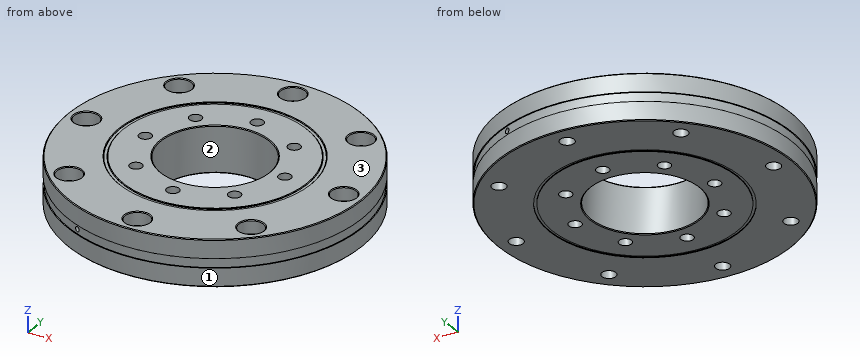
from build123d import *

# Parameters (mm, degrees)
BOSS_EXTRUDE1_DEPTH          = 7.5
BOSS_EXTRUDE1_DEPTH_BACK     = 7.5
SKETCH4_R                    = 2
CIRPATTERN1_COUNT            = 8
BOSS_EXTRUDE4_DEPTH          = 7.5
BOSS_EXTRUDE4_DEPTH_BACK     = 7.5
SKETCH9_R                    = 47.5
SKETCH9_R_2                  = 17.5
SKETCH10_R                   = 4
CUT_EXTRUDE1_DEPTH           = 4.4
SKETCH11_R                   = 2.25
CUT_EXTRUDE2_DEPTH           = 69.82949949
CHAMFER2_SIZE                = 0.25
CHAMFER1_SIZE                = 0.25
CIRPATTERN2_COUNT            = 8
CHAMFER2_OF_CIRPATTERN2_SIZE = 0.25
SKETCH12_W                   = 0.25
SKETCH12_H                   = 0.9
SKETCH12_W_2                 = 3
SKETCH12_H_2                 = 0.3
SKETCH13_W                   = 0.825
SKETCH13_H                   = 17.2
CIRPATTERN3_COUNT            = 2
CHAMFER3_SIZE                = 0.2


with BuildPart() as part:
    # Sketch4 → Boss-Extrude1 (new, two sides: drawn at the far end of the back side and taken through both)
    with BuildSketch(Plane.XY.offset(-BOSS_EXTRUDE1_DEPTH_BACK)):
        with Locations((0, 22.5)):
            Circle(SKETCH4_R)
    extrude(amount=BOSS_EXTRUDE1_DEPTH + BOSS_EXTRUDE1_DEPTH_BACK)

    # Boss-Extrude2 cone 1 section (through the dimple's axis) → Boss-Extrude2 (revolve)
    with BuildSketch(Plane(origin=(0, 22.5, 7.5), x_dir=(0, -1, 0), z_dir=(1, 0, 0))):
        Polygon((0, 0), (2, 0), (0, 2), align=None)
    revolve(axis=Axis((0, 22.5, 7.5), (0, 0, -1)))

    # Boss-Extrude3 cone 1 section (through the dimple's axis) → Boss-Extrude3 (revolve)
    with BuildSketch(Plane(origin=(0, 22.5, -7.5), x_dir=(0, 1, 0), z_dir=(1, 0, 0))):
        Polygon((0, 0), (2, 0), (0, 2), align=None)
    revolve(axis=Axis((0, 22.5, -7.5), (0, 0, 1)))


with BuildPart() as cirpattern1_1:
    # CirPattern1: pattern copy
    add(part.part.rotate(Axis((0, 0, 0), (0, 0, 1)), 1 * 360 / CIRPATTERN1_COUNT))


with BuildPart() as cirpattern1_2:
    # CirPattern1: pattern copy
    add(part.part.rotate(Axis((0, 0, 0), (0, 0, 1)), 2 * 360 / CIRPATTERN1_COUNT))


with BuildPart() as cirpattern1_3:
    # CirPattern1: pattern copy
    add(part.part.rotate(Axis((0, 0, 0), (0, 0, 1)), 3 * 360 / CIRPATTERN1_COUNT))


with BuildPart() as cirpattern1_4:
    # CirPattern1: pattern copy
    add(part.part.rotate(Axis((0, 0, 0), (0, 0, 1)), 4 * 360 / CIRPATTERN1_COUNT))


with BuildPart() as cirpattern1_5:
    # CirPattern1: pattern copy
    add(part.part.rotate(Axis((0, 0, 0), (0, 0, 1)), 5 * 360 / CIRPATTERN1_COUNT))


with BuildPart() as cirpattern1_6:
    # CirPattern1: pattern copy
    add(part.part.rotate(Axis((0, 0, 0), (0, 0, 1)), 6 * 360 / CIRPATTERN1_COUNT))


with BuildPart() as cirpattern1_7:
    # CirPattern1: pattern copy
    add(part.part.rotate(Axis((0, 0, 0), (0, 0, 1)), 7 * 360 / CIRPATTERN1_COUNT))


with BuildPart() as body_9:
    # Sketch9 → Boss-Extrude4 (new, two sides: drawn at the far end of the back side and taken through both)
    with BuildSketch(Plane.XY.offset(-BOSS_EXTRUDE4_DEPTH_BACK)):
        Circle(SKETCH9_R)
        Circle(SKETCH9_R_2, mode=Mode.SUBTRACT)
    extrude(amount=BOSS_EXTRUDE4_DEPTH + BOSS_EXTRUDE4_DEPTH_BACK)

    # Combine1: cut CirPattern1_3, CirPattern1_1, CirPattern1_2, part, CirPattern1_6, CirPattern1_5, CirPattern1_4, CirPattern1_7
    add(cirpattern1_3.part, mode=Mode.SUBTRACT)
    add(cirpattern1_1.part, mode=Mode.SUBTRACT)
    add(cirpattern1_2.part, mode=Mode.SUBTRACT)
    add(part.part, mode=Mode.SUBTRACT)
    add(cirpattern1_6.part, mode=Mode.SUBTRACT)
    add(cirpattern1_5.part, mode=Mode.SUBTRACT)
    add(cirpattern1_4.part, mode=Mode.SUBTRACT)
    add(cirpattern1_7.part, mode=Mode.SUBTRACT)

    # Sketch10 → Cut-Extrude1 (cut)
    with BuildSketch(Plane.XY.offset(7.5)):
        with Locations((0, 41.5)):
            Circle(SKETCH10_R)
    cut_extrude1 = extrude(amount=-CUT_EXTRUDE1_DEPTH, mode=Mode.SUBTRACT)

    # Sketch11 → Cut-Extrude2 (cut, through all)
    with BuildSketch(Plane.XY.offset(7.5)):
        with Locations((0, 41.5)):
            Circle(SKETCH11_R)
    cut_extrude2 = extrude(amount=-CUT_EXTRUDE2_DEPTH, mode=Mode.SUBTRACT)

    # Chamfer2
    chamfer2_edges = [body_9.edges().sort_by_distance(p)[0] for p in [
        (-4, 41.5, 7.5),
    ]]
    chamfer(chamfer2_edges, length=CHAMFER2_SIZE)

    # Chamfer1
    chamfer1_edges = [body_9.edges().sort_by_distance(p)[0] for p in [
        (-47.5, 0, -7.5),
        (-17.5, 0, -7.5),
        (-47.5, 0, 7.5),
        (-17.5, 0, 7.5),
    ]]
    chamfer(chamfer1_edges, length=CHAMFER1_SIZE)

    # CirPattern2: Cut-Extrude1, Cut-Extrude2 ×8 about axis
    cirpattern2_axis = Axis((0, 0, 0), (0, 0, 1))
    add([cut_extrude1.rotate(cirpattern2_axis, i * 360 / CIRPATTERN2_COUNT) for i in range(1, CIRPATTERN2_COUNT)], mode=Mode.SUBTRACT)
    add([cut_extrude2.rotate(cirpattern2_axis, i * 360 / CIRPATTERN2_COUNT) for i in range(1, CIRPATTERN2_COUNT)], mode=Mode.SUBTRACT)

    # Chamfer2 of CirPattern2
    chamfer2_of_cirpattern2_edges = [body_9.edges().sort_by_distance(p)[0] for p in [
        (-32.173358544, 26.516504294, 7.5),
        (-41.5, -4, 7.5),
        (-26.516504294, -32.173358544, 7.5),
        (4, -41.5, 7.5),
        (32.173358544, -26.516504294, 7.5),
        (41.5, 4, 7.5),
        (26.516504294, 32.173358544, 7.5),
    ]]
    chamfer(chamfer2_of_cirpattern2_edges, length=CHAMFER2_OF_CIRPATTERN2_SIZE)

    # Sketch12 → Cut-Revolve1 (revolve, cut)
    with BuildSketch(Plane(origin=(0, 0, 0), x_dir=(0, 0, -1), z_dir=(1, 0, 0)), mode=Mode.PRIVATE) as cut_revolve1_sk:
        with Locations((-7.375, 30.3)):
            Rectangle(SKETCH12_W, SKETCH12_H)
        with Locations((7.375, 30.3)):
            Rectangle(SKETCH12_W, SKETCH12_H)
        with Locations((0, 47.35)):
            Rectangle(SKETCH12_W_2, SKETCH12_H_2)
    revolve(cut_revolve1_sk.sketch.rotate(Axis((0, 0, 7.5), (0, 0, -1)), 90), axis=Axis((0, 0, 7.5), (0, 0, -1)), mode=Mode.SUBTRACT)

    # Sketch13 → Cut-Revolve2 (revolve, cut)
    with BuildSketch(Plane(origin=(0, 0, 0), x_dir=(0, 0, -1), z_dir=(0.9238795325112865, -0.3826834323650906, 0)), mode=Mode.PRIVATE) as cut_revolve2_sk:
        with Locations((-0.4125, 38.9)):
            Rectangle(SKETCH13_W, SKETCH13_H)
    cut_revolve2 = revolve(cut_revolve2_sk.sketch.rotate(Axis((11.854473416, 28.619230496, 0), (-0.3826834323650891, -0.9238795325112871, 0)), 90), axis=Axis((11.854473416, 28.619230496, 0), (-0.3826834323650891, -0.9238795325112871, 0)), mode=Mode.SUBTRACT)

    # CirPattern3: Cut-Revolve2 ×2 about axis
    cirpattern3_axis = Axis((0, 0, 7.5), (0, 0, -1))
    for i in range(1, CIRPATTERN3_COUNT):
        add(cut_revolve2.rotate(cirpattern3_axis, i * 360 / CIRPATTERN3_COUNT), mode=Mode.SUBTRACT)

    # Chamfer3
    chamfer3_edges = [body_9.edges().sort_by_distance(p)[0] for p in [
        (-30.75, 0, 7.5),
        (-29.85, 0, 7.5),
    ]]
    chamfer(chamfer3_edges, length=CHAMFER3_SIZE)


solid = body_9.part
Could you check a few things on this model? Use its own coordinates, in mm. Face numbers are marked on the shaded views. Round coordinates to 2 decimals unless told otherwise and drop trailing zeros. Use a Markdown table: item, result.
1. If we section it at A-A (y = 0): State how many separate pieces and enclosed holes the cut face has, then the cut area to 3 significant figures.
Answer key:
| item | result |
|---|---|
| separate pieces | 6 |
| enclosed holes | 0 |
| area | 611 mm^2 |
2. Please list where these lines run through material, in increasing order: probe 1 along Y at (x, z) = (0, 4.6); probe 2 along Y at (x, z) = (-15.5, -5.75); probe 3 along Z at (x, y) = (-27, 28).
Answer key:
| item | result |
|---|---|
| probe 1 | y = -47.5 to -45.5, -37.5 to -24.5, -20.5 to -17.5, 17.5 to 20.5, 24.5 to 37.5, 45.5 to 47.5 |
| probe 2 | y = -44.9 to -17.87, -13.95 to -8.12, 8.12 to 13.95, 17.87 to 44.9 |
| probe 3 | z = -7.5 to 3.1 |
3. We'd pull the mould along Y, two halves only. Please class the marked faces 1, 2 and 3: +Y half, -Y half, draft (parallel to the pull), parting line (faces both ways), or undercut.
Answer key:
| item | result |
|---|---|
| face 1 | parting line |
| face 2 | undercut |
| face 3 | draft |
4. For pin 1 Ø2.5 at (x, y) = (-0.5, -41.5) entering from +Z; pin 2 Ø6.5 at (x, y) = (-39.5, 0) entering from +Z; pin 3 Ø2 at (y, z) = (-37, -4) entering from +X; pin 4 Ø2 at (x, z) = (-30, 4.5) entering from +Y, each with a flat end and sliding along its axis, tell me the tip position at first contact or that it passes through.
Answer key:
| item | result |
|---|---|
| pin 1 | passes through |
| pin 2 | stops at z = 7.5 |
| pin 3 | stops at x = 30.99 |
| pin 4 | stops at y = 37.62 |
